CAD build for the part. Positions are in the model's coordinates, mm. Round coordinates to 2 decimals unless told otherwise and drop trailing zeros. Loops run counter-clockwise (first coordinate to the right, second up) from the corner with the lowest first, then second, coordinate; pieces in that order, holes last.
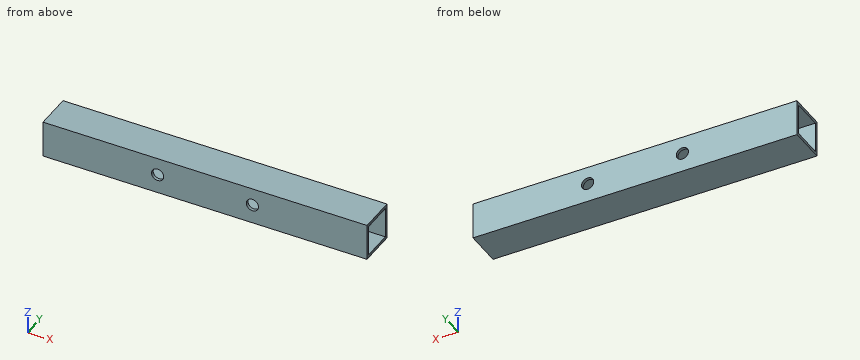
from build123d import *

# Parameters (mm, degrees)
SKETCH1_W           = 106
SKETCH1_H           = 12
BOSS_EXTRUDE1_DEPTH = 12
SKETCH2_R           = 2
CUT_EXTRUDE1_DEPTH  = 12
SKETCH3_W           = 10
SKETCH3_H           = 10
CUT_EXTRUDE2_DEPTH  = 128


with BuildPart() as part:
    # Sketch1 → Boss-Extrude1 (new body)
    with BuildSketch(Plane.XY):
        Rectangle(SKETCH1_W, SKETCH1_H)
    extrude(amount=BOSS_EXTRUDE1_DEPTH)

    # Sketch2 → Cut-Extrude1 (cut)
    with BuildSketch(Plane(origin=(0, 6, 0), x_dir=(1, 0, 0), z_dir=(0, 1, 0))):
        with Locations((-15.5, -6.282258571)):
            Circle(SKETCH2_R)
        with Locations((15.5, -6.282258571)):
            Circle(SKETCH2_R)
    extrude(amount=-CUT_EXTRUDE1_DEPTH, mode=Mode.SUBTRACT)

    # Sketch3 → Cut-Extrude2 (cut)
    with BuildSketch(Plane(origin=(53, 0, 0), x_dir=(0, 0, -1), z_dir=(1, 0, 0))):
        with Locations((-6, 0)):
            Rectangle(SKETCH3_W, SKETCH3_H)
    extrude(amount=-CUT_EXTRUDE2_DEPTH, mode=Mode.SUBTRACT)


solid = part.part
Item 1: Cut at C-C (z = 3). List the corners of the cut face in (x, y), plus the area to 3 significant figures.
Verdict:
outline: (-53, -6) - (53, -6) - (53, -5) - (-53, -5) - close; (-53, 5) - (53, 5) - (53, 6) - (-53, 6) - close
area: 212 mm2
Item 2: Cut at B-B (x = 15.5). List the corners of the cut face in (y, z).
Verdict:
outline: (-6, 0) - (6, 0) - (6, 4.28) - (5, 4.28) - (5, 1) - (-5, 1) - (-5, 4.28) - (-6, 4.28) - close; (-6, 8.28) - (-5, 8.28) - (-5, 11) - (5, 11) - (5, 8.28) - (6, 8.28) - (6, 12) - (-6, 12) - close
Item 3: Wall check: L1, parallel to Z at x = 41, y = -2; L2, parallel to Y at x = -47.5, z = 7.25; L3, parallel to Z at x = -15.5, y = 5.25. Give the ranges that are in metal, low to high.
Verdict:
L1: z = 0 to 1, 11 to 12
L2: y = -6 to -5, 5 to 6
L3: z = 0 to 4.28, 8.28 to 12
Item 4: Cut at A-A (y = 4). List the corners of the cut face in (x, z).
Verdict:
outline: (-53, 0) - (53, 0) - (53, 1) - (-53, 1) - close; (-53, 11) - (53, 11) - (53, 12) - (-53, 12) - close
Item 5: Flat gauge pin, fed straight in: P1, Ø3, axis at x = 15.5, z = 6.28, coming from the +Y side. Where does the tip first touch, or does it go through?
Verdict:
P1: passes through
